Design review of the part built by this model. Coordinates are the model's own, in mm. Round coordinates to 2 decimals unless told otherwise and drop trailing zeros. Loops run counter-clockwise (first coordinate to the right, second up) from the corner with the lowest first, then second, coordinate; pieces in that order, holes last. Notation, with made-up numbers: (75, 30) - (131, 30) arc R7 ccw to (131, 39) - close; hole circle Ø8 at (-22.5, 47). An arc over 180 degrees is marked (long way). Return JSON: item names as keys, results as strings. Group by question number.
(1) We need section B-B, the plane z = 2.3. Give the number of separate pieces and of enclosed holes in the cut face, and give its area (3 significant figures).
(2) We need section A-A, the plane x = 19. Write out the cut boundary in (y, z), and give its area (3 significant figures).
(3) We need section C-C, the plane x = -57.5. Write out the cut boundary in (y, z), and give its area (3 significant figures).
(4) Wall thickness on L1, parallel to Y at x = -38.05, z = 1.05; L2, parallel to Y at x = 57.5, z = 1.9; L3, parallel to Y at x = -63.15, z = 1.3: over which ranges is each line inside the solid? List them lowest first. Write a range as [from, to].
(5) We need section D-D, the plane y = 28. Write out the cut boundary in (x, z), and give its area (3 significant figures).
(6) Clearance check with flat-ended pins moving along their axes: pin 1 (2 mm diameter, centred on x = 38.05, y = 13.55, fed in from +Z); pin 2 (0.9 mm diameter, centred on x = -56, z = 1, fed in from -Y); pin 3 (0.9 mm diameter, centred on x = -57, z = 2, fed in from +Y). State where each tip first meets the part, or that it passes through.
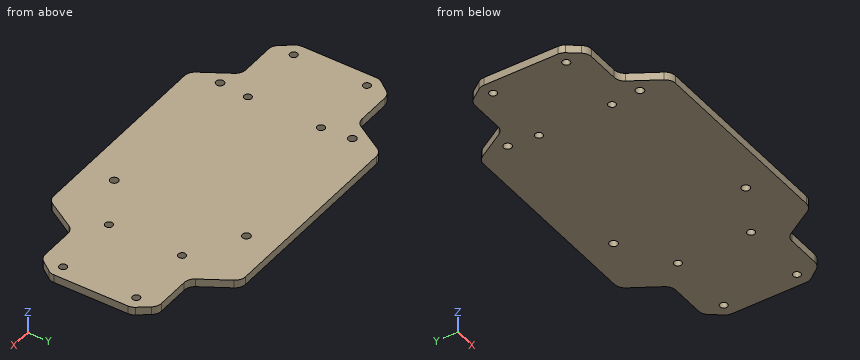
from build123d import *

# Parameters (mm, degrees)
SKETCH1_R           = 1.4
SKETCH1_R_2         = 1.5
BOSS_EXTRUDE1_DEPTH = 3


with BuildPart() as part:
    # Sketch1 → Boss-Extrude1 (new body)
    with BuildSketch(Plane.XY):
        with BuildLine():
            Line((68, -13.680285878), (68, 13.680285878))
            ThreePointArc((68, 13.680285878), (67.79859538, 14.93355087), (67.21466343, 16.060609182))
            Line((67.21466343, 16.060609182), (64.349302592, 19.930323303))
            ThreePointArc((64.349302592, 19.930323303), (62.93445954, 21.122204726), (61.134639162, 21.55))
            Line((61.134639162, 21.55), (48.7578418, 21.55))
            ThreePointArc((48.7578418, 21.55), (46.79161141, 22.066619738), (45.333277733, 23.483030974))
            Line((45.333277733, 23.483030974), (39.216722267, 33.616969026))
            ThreePointArc((39.216722267, 33.616969026), (37.75838859, 35.033380262), (35.7921582, 35.55))
            Line((35.7921582, 35.55), (-35.7921582, 35.55))
            ThreePointArc((-35.7921582, 35.55), (-37.75838859, 35.033380262), (-39.216722267, 33.616969026))
            Line((-39.216722267, 33.616969026), (-45.333277733, 23.483030974))
            ThreePointArc((-45.333277733, 23.483030974), (-46.79161141, 22.066619738), (-48.7578418, 21.55))
            Line((-48.7578418, 21.55), (-61.134639162, 21.55))
            ThreePointArc((-61.134639162, 21.55), (-62.93445954, 21.122204726), (-64.349302592, 19.930323303))
            Line((-64.349302592, 19.930323303), (-67.21466343, 16.060609182))
            ThreePointArc((-67.21466343, 16.060609182), (-67.79859538, 14.93355087), (-68, 13.680285878))
            Line((-68, 13.680285878), (-68, -13.680285878))
            ThreePointArc((-68, -13.680285878), (-67.79859538, -14.93355087), (-67.21466343, -16.060609182))
            Line((-67.21466343, -16.060609182), (-64.349302592, -19.930323303))
            ThreePointArc((-64.349302592, -19.930323303), (-62.93445954, -21.122204726), (-61.134639162, -21.55))
            Line((-61.134639162, -21.55), (-48.7578418, -21.55))
            ThreePointArc((-48.7578418, -21.55), (-46.79161141, -22.066619738), (-45.333277733, -23.483030974))
            Line((-45.333277733, -23.483030974), (-39.216722267, -33.616969026))
            ThreePointArc((-39.216722267, -33.616969026), (-37.75838859, -35.033380262), (-35.7921582, -35.55))
            Line((-35.7921582, -35.55), (35.7921582, -35.55))
            ThreePointArc((35.7921582, -35.55), (37.75838859, -35.033380262), (39.216722267, -33.616969026))
            Line((39.216722267, -33.616969026), (45.333277733, -23.483030974))
            ThreePointArc((45.333277733, -23.483030974), (46.79161141, -22.066619738), (48.7578418, -21.55))
            Line((48.7578418, -21.55), (61.134639162, -21.55))
            ThreePointArc((61.134639162, -21.55), (62.93445954, -21.122204726), (64.349302592, -19.930323303))
            Line((64.349302592, -19.930323303), (67.21466343, -16.060609182))
            ThreePointArc((67.21466343, -16.060609182), (67.79859538, -14.93355087), (68, -13.680285878))
        make_face()
        with Locations((38.05, -13.55)):
            Circle(SKETCH1_R, mode=Mode.SUBTRACT)
        with Locations((63.15, -13.55)):
            Circle(SKETCH1_R, mode=Mode.SUBTRACT)
        with Locations(Location((63.15, 13.55, 0), (0, 0, 180))):
            Circle(SKETCH1_R, mode=Mode.SUBTRACT)
        with Locations(Location((38.05, 13.55, 0), (0, 0, 180))):
            Circle(SKETCH1_R, mode=Mode.SUBTRACT)
        with Locations(Location((-38.05, -13.55, 0), (0, 0, 180))):
            Circle(SKETCH1_R, mode=Mode.SUBTRACT)
        with Locations(Location((-63.15, -13.55, 0), (0, 0, 180))):
            Circle(SKETCH1_R, mode=Mode.SUBTRACT)
        with Locations((-63.15, 13.55)):
            Circle(SKETCH1_R, mode=Mode.SUBTRACT)
        with Locations((-38.05, 13.55)):
            Circle(SKETCH1_R, mode=Mode.SUBTRACT)
        with Locations((-39, 24.5)):
            Circle(SKETCH1_R_2, mode=Mode.SUBTRACT)
        with Locations((19, 24.5)):
            Circle(SKETCH1_R_2, mode=Mode.SUBTRACT)
        with Locations(Location((19, -24.5, 0), (0, 0, 180))):
            Circle(SKETCH1_R_2, mode=Mode.SUBTRACT)
        with Locations(Location((-39, -24.5, 0), (0, 0, 180))):
            Circle(SKETCH1_R_2, mode=Mode.SUBTRACT)
    extrude(amount=BOSS_EXTRUDE1_DEPTH)


solid = part.part
Solutions:
{
 "1": {"separate pieces": "1", "enclosed holes": "12", "area": "8,080 mm^2"},
 "2": {"outline": "(-35.55, 0) - (-26, 0) - (-26, 3) - (-35.55, 3) - close; (-23, 0) - (23, 0) - (23, 3) - (-23, 3) - close; (26, 0) - (35.55, 0) - (35.55, 3) - (26, 3) - close", "area": "195 mm^2"},
 "3": {"outline": "(-21.55, 0) - (21.55, 0) - (21.55, 3) - (-21.55, 3) - close", "area": "129 mm^2"},
 "4": {"L1": "[-34.85, -25.66], [-23.34, -14.95], [-12.15, 12.15], [14.95, 23.34], [25.66, 34.85]", "L2": "[-21.55, 21.55]", "L3": "[-21.01, -14.95], [-12.15, 12.15], [14.95, 21.01]"},
 "5": {"outline": "(-42.61, 0) - (42.61, 0) - (42.61, 3) - (-42.61, 3) - close", "area": "256 mm^2"},
 "6": {"pin 1": "through", "pin 2": "y = -21.55", "pin 3": "y = 21.55"}
}
